Read the model definition and answer for the solid it produces. Units are mm, in the model's axes. A direction names the side the tool comes from. Give positions to 0.01 mm unless a question says otherwise; leave off trailing zeros. Order: outer loops, then holes, each group sorted by start corner. A loop starts at its lowest first (then second) coordinate and runs counter-clockwise, first axis right, second up. Notation, with made-up numbers: (25.5, 72.25) - (50.5, 72.25) arc R13 ccw to (50.5, 78.25) - close; hole circle Ø5 at (-26, 10.5). An arc over 180 degrees is marked (long way). Return JSON: item names as keys, results as strings.
Autodesk Inventor part; units mm, degrees
ref_plane "YZ Plane" through (0, 0, 0) normal (1, 0, 0) x (0, 1, 0)
ref_plane "XZ Plane" through (0, 0, 0) normal (0, 1, 0) x (-1, 0, 0)
ref_plane "XY Plane" through (0, 0, 0) normal (0, 0, 1) x (1, 0, 0)
sketch "Sketch4" plane through (0, 0, 0) normal (0, 0, 1) x (1, 0, 0)
  line L0 (0, 0) -> (12, 0)
  line L1 (12, 0) -> (12, -10)
  line L2 (12, -10) -> (27, -10)
  line L3 (27, -10) -> (27, 0)
  line L4 (27, 0) -> (39, 0)
  line L5 (0, -3) -> (9, -3)
  line L6 (9, -3) -> (9, -13)
  line L7 (9, -13) -> (30, -13)
  line L8 (30, -13) -> (30, -3)
  line L9 (30, -3) -> (39, -3)
  line L10 (0, -3) -> (0, 0)
  line L11 (39, -3) -> (39, 0)
  dimension "d14" = 12
  dimension "d15" = 12
  dimension "d16" = 10
  dimension "d17" = 15
  dimension "d18" = 3
extrude "Extrusion4" add sketch "Sketch4" along normal blind 30
sketch "Sketch5" plane through (0, 0, 0) normal (0, 1, 0) x (1, 0, 0)
  line L0 (9, 0) -> (0, 0) construction
  line L1 (9, 0) -> (9, -30) construction
  line L2 (0, -30) -> (9, -30) construction
  line L3 (0, 0) -> (0, -30) construction
  line L4 (39, 0) -> (30, 0) construction
  line L5 (39, 0) -> (39, -30) construction
  line L6 (30, -30) -> (39, -30) construction
  line L7 (30, 0) -> (30, -30) construction
  circle A0 centre (4.5, -22.5) radius 2.5
  circle A1 centre (4.5, -7.5) radius 2.5
  line L8 (4.5, -22.5) -> (4.5, -7.5) construction
  line L9 (19.5, -30) -> (19.5, 0)
  line L10 (12, 0) -> (27, 0)
  line L11 (27, -30) -> (12, -30)
  circle A2 centre (34.5, -22.5) radius 2.5
  circle A3 centre (34.5, -7.5) radius 2.5
  line L12 (34.5, -22.5) -> (34.5, -7.5) construction
  point P0 (4.5, -30)
  point P1 (4.5, 0)
  point P2 (4.5, -15)
  point P3 (0, -15)
  point P4 (34.5, -15)
  dimension "d21" = 5
  dimension "d22" = 5
  dimension "d23" = 15
extrude "Extrusion5" cut sketch "Sketch5" against normal through all
sketch "Sketch6" plane through (9, -13, 0) normal (0, -1, 0) x (1, 0, 0)
  line L0 (3, 30) -> (-9, 30)
  line L1 (30, 0) -> (30, 30)
  line L2 (-9, 30) -> (30, 30)
  line L3 (30, 30) -> (30, 15)
  line L4 (30, 15) -> (-9, 15)
  line L5 (-9, 15) -> (-9, 30)
  point P0 (-9, 0)
extrude "Extrusion6" cut sketch "Sketch6" against normal through all
sketch "Sketch7" plane through (9, -13, 0) normal (0, -1, 0) x (1, 0, 0)
  circle A0 centre (10.5, 11.7) radius 2.5
  circle A1 centre (10.5, 4.2) radius 2.5
  line L0 (10.5, 4.2) -> (10.5, 11.7) construction
  line L1 (21, 15) -> (0, 15)
  point P0 (-9, 0)
  point P1 (10.5, 15)
  dimension "d28" = 5
  dimension "d29" = 5
  dimension "d30" = 7.5
  dimension "d31" = 3.3
extrude "Extrusion7" cut sketch "Sketch7" against normal through all
sketch "Sketch8" plane through (0, 0, 0) normal (0, 1, 0) x (1, 0, 0)
  line L0 (27, -15) -> (39, -15)
  line L1 (0, 0) -> (39, 0)
  line L2 (39, 0) -> (39, -15)
  line L3 (39, -15) -> (0, -15)
  line L4 (0, -15) -> (0, 0)
  circle A0 centre (4.5, -7.5) radius 2.5
  circle A1 centre (34.5, -7.5) radius 2.5
extrude "Extrusion8" add sketch "Sketch8" along normal blind 4
sketch "Sketch9" plane through (0, 0, 0) normal (0, -1, 0) x (1, 0, 0)
  line L0 (9, 15) -> (0, 15)
  line L1 (0, 0) -> (0, 15)
  line L2 (9, 0) -> (0, 0)
  line L3 (9, 0) -> (9, 15)
  circle A0 centre (4.5, 7.5) radius 2.5
  line L4 (39, 15) -> (30, 15)
  line L5 (30, 0) -> (30, 15)
  line L6 (39, 0) -> (30, 0)
  line L7 (39, 0) -> (39, 15)
  circle A1 centre (34.5, 7.5) radius 2.5
extrude "Extrusion9" cut sketch "Sketch9" along normal through all
chamfer "Chamfer1" distance 2 angle 45 4 edges at (9, -6.5, 15) (30, -6.5, 15) (30, -6.5, 0) (9, -6.5, 0)
chamfer "Chamfer2" distance 2 angle 45 4 edges at (39, 2, 15) (39, 2, 0) (0, 2, 0) (0, 2, 15)
equation "\"d15\" = d14"
properties part number "WA03" material "ABS Plastic"
Q1. For faces 1 (the flat face through (9, -6, 7)), 2 (the cylindrical face through (17, -11.5, 11.8)), 3 (the flat face through (19, -10, 7)), determine the directions among +Z, -Z, +X, -X, +Y, -Y from which every point of the face is accessible in a straight line to the end or side of a thin tool.
Values:
{"face 1": "+Z, -Z, -X, -Y", "face 2": "-Y", "face 3": "+Z, -Z"}
Q2. A cutting plane is placed at C-C (x = 19.5). Write down the section's boundary in (y, z).
Values:
{"outline": "(-13, 0) - (-10, 0) - (-10, 1.7) - (-13, 1.7) - close; (-13, 6.7) - (-10, 6.7) - (-10, 9.2) - (-13, 9.2) - close; (-13, 14.2) - (-10, 14.2) - (-10, 15) - (-13, 15) - close; (0, 0) - (4, 0) - (4, 15) - (0, 15) - close"}
Q3. A cutting plane is placed at A-A (y = -9.5). Write down the section's boundary in (x, z), and give its area (3 significant figures).
Values:
{"outline": "(9, 2) - (11, 0) - (12, 0) - (12, 15) - (11, 15) - (9, 13) - close; (27, 0) - (28, 0) - (30, 2) - (30, 13) - (28, 15) - (27, 15) - close", "area": "82.0 mm²"}
Q4. Determine the mould class of faces 4 (the flat face through (20, 1, 15)), 5 (the flat face through (29, -7, 1)), 6 (the cylindrical face through (17, -11.5, 4.3)), 7 (the flat face through (27, -5, 7)) for opening direction Z: released by +Z, released by -Z, zero draft, split by the parting line, or undercut.
Values:
{"face 4": "released by +Z", "face 5": "released by -Z", "face 6": "undercut", "face 7": "zero draft"}
Q5. A cutting plane is placed at B-B (x = 34.5). Write down the section's boundary in (y, z), and give its area (3 significant figures).
Values:
{"outline": "(0, 0) - (4, 0) - (4, 5) - (0, 5) - close; (0, 10) - (4, 10) - (4, 15) - (0, 15) - close", "area": "40.0 mm²"}
Q6. Given pin 1 (1.5 mm diameter, centred on x = 7, y = -5, fed in from +Z); pin 2 (5.5 mm diameter, centred on x = 6.5, z = 4.5, fed in from -Y); pin 3 (3 mm diameter, centred on x = 19.5, z = 4.2, fed in from -Y); pin 4 (5.5 mm diameter, centred on y = -9, z = 7.5, fed in from -X), each flat-ended and moving along its own axis, determine where each tip first touches the part or whether it passes through.
Values:
{"pin 1": "passes through", "pin 2": "stops at y = -13", "pin 3": "stops at y = 0", "pin 4": "stops at x = 9"}
Q7. Consider L1, parallel to Z at x = 19.5, y = -11.4; L2, parallel to X at y = -4.75, z = 9.25; L3, parallel to Z at x = 34.5, y = 2.9. Determine where each line is inside the solid, lowest interval first.
Values:
{"L1": "z = 0 to 1.7, 6.7 to 9.2, 14.2 to 15", "L2": "x = 9 to 12, 27 to 30", "L3": "z = 0 to 5, 10 to 15"}
Q8. A cutting plane is placed at D-D (z = 4.2). Write down the section's boundary in (x, y), and give its area (3 significant figures).
Values:
{"outline": "(0, 0) - (9, 0) - (9, -13) - (17, -13) - (17, -10) - (12, -10) - (12, 0) - (27, 0) - (27, -10) - (22, -10) - (22, -13) - (30, -13) - (30, 0) - (39, 0) - (39, 4) - (0, 4) - close", "area": "264 mm²"}
